```python
from build123d import *

# Parameters (mm, degrees)
F0_R     = 3.9751
F0_R_2   = 15.875
F0_R_3   = 3.96875
F1_DEPTH = 19.05
F3_DEPTH = 9.525
F5_R     = 9.525
F5_R_2   = 3.9751
F5_R_3   = 3.96875
F6_DEPTH = 2.54


# Not quite as in the source:
# - a feature of the source that left no trace in its solid (it failed there, or was rolled back) is left out


with BuildPart() as f1:
    # F0 (on Top) → F1 (new body)
    with BuildSketch(Plane.XY):
        with BuildLine():
            Line((-68.2625, -74.6125), (68.2625, -74.6125))
            ThreePointArc((68.2625, -74.6125), (72.7526280605, -72.7526280605), (74.6125, -68.2625))
            Line((74.6125, -68.2625), (74.6125, -4.7625))
            Line((74.6125, -4.7625), (15.1437848225, -4.7625))
            ThreePointArc((15.1437848225, -4.7625), (-15.875, 0), (15.1437848225, 4.7625))
            Line((15.1437848225, 4.7625), (74.6125, 4.7625))
            Line((74.6125, 4.7625), (74.6125, 68.2625))
            ThreePointArc((74.6125, 68.2625), (72.7526280605, 72.7526280605), (68.2625, 74.6125))
            Line((68.2625, 74.6125), (-68.2625, 74.6125))
            ThreePointArc((-68.2625, 74.6125), (-72.7526280605, 72.7526280605), (-74.6125, 68.2625))
            Line((-74.6125, 68.2625), (-74.6125, -68.2625))
            ThreePointArc((-74.6125, -68.2625), (-72.7526280605, -72.7526280605), (-68.2625, -74.6125))
        make_face()
        with Locations((-55.5625, -55.5625)):
            Circle(F0_R, mode=Mode.SUBTRACT)
        with Locations((-30.1625, -30.1625)):
            Circle(F0_R_2, mode=Mode.SUBTRACT)
        with Locations((55.5625, -55.5625)):
            Circle(F0_R, mode=Mode.SUBTRACT)
        with Locations((30.1625, -30.1625)):
            Circle(F0_R_2, mode=Mode.SUBTRACT)
        with Locations((-30.1625, 30.1625)):
            Circle(F0_R_2, mode=Mode.SUBTRACT)
        with Locations((-55.5625, 55.5625)):
            Circle(F0_R_3, mode=Mode.SUBTRACT)
        with Locations((30.1625, 30.1625)):
            Circle(F0_R_2, mode=Mode.SUBTRACT)
        with Locations((55.5625, 55.5625)):
            Circle(F0_R, mode=Mode.SUBTRACT)
    extrude(amount=F1_DEPTH)

    # F2 (on face) → F3 (join)
    with BuildSketch(Plane(origin=(0, 0, 0), x_dir=(1, 0, 0), z_dir=(0, 0, -1))):
        with BuildLine():
            Line((74.6125, 4.7625), (15.1437848225, 4.7625))
            ThreePointArc((15.1437848225, 4.7625), (15.875, 0), (15.1437848225, -4.7625))
            Line((15.1437848225, -4.7625), (74.6125, -4.7625))
            Line((74.6125, -4.7625), (74.6125, 4.7625))
        make_face()
    extrude(amount=-F3_DEPTH)

    # F5 (on face) → F6 (cut)
    with BuildSketch(Plane.XY.offset(19.05)):
        with Locations((-55.5625, -55.5625)):
            Circle(F5_R)
        with Locations((-55.5625, -55.5625)):
            Circle(F5_R_2, mode=Mode.SUBTRACT)
        with Locations((55.5625, -55.5625)):
            Circle(F5_R)
        with Locations((55.5625, -55.5625)):
            Circle(F5_R_2, mode=Mode.SUBTRACT)
        with Locations((55.5625, 55.5625)):
            Circle(F5_R)
        with Locations((55.5625, 55.5625)):
            Circle(F5_R_2, mode=Mode.SUBTRACT)
        with Locations((-55.5625, 55.5625)):
            Circle(F5_R)
        with Locations((-55.5625, 55.5625)):
            Circle(F5_R_3, mode=Mode.SUBTRACT)
    extrude(amount=-F6_DEPTH, mode=Mode.SUBTRACT)


solid = f1.part
```
Work out the finished part from the listing and answer in its coordinate system (mm). A direction names the side the tool comes from. Give positions to 0.01 mm unless a question says otherwise; leave off trailing zeros. Write item = value, one per line.
Q1. Flat-ended cylindrical pins translate along their axes: pin 1 Ø9 at (x, y) = (55.56, 55.56) entering from +Z; pin 2 Ø4 at (x, y) = (-39.5, -12) entering from -Z. Find the tip coordinate at first contact, or state that the pin passes through.
Computed values:
pin_1 = 16.51
pin_2 = 0
Q2. Section C-C on z = 3.5 is taken. State how many separate pieces and enclosed holes the cut face has, and give its area (3 significant figures).
Computed values:
separate_pieces = 1
enclosed_holes = 9
area = 18,100 mm^2
Q3. For a pull along Y with two mould halves and no side action, classify faces 1 (the flat face through (-1, -74.612, 9)), 2 (the cylindrical face through (18.46, 40.89, 9.39)), 3 (the flat face through (1, 74.612, 9)), 4 (the flat face through (-18, 1, 19.05)) as pulls with the +Y half, pulls with the -Y half, needs draft (parallel to the pull), parting line crosses it, or undercut.
Computed values:
face_1 = pulls with the -Y half
face_2 = undercut
face_3 = pulls with the +Y half
face_4 = needs draft
Q4. A tool of negligible diameter and unlimited length cuts with its end or side. For faces 5 (the flat face through (-51, 56, 16.51)), 6 (the flat face through (45, -4.762, 14)), 7 (the cylindrical face through (-72.703, 72.802, 9.392)), from which of +Z, -Z, +X, -X, +Y, -Y can it reach the whole face along a straight path? Write none if from no direction.
Computed values:
face_5 = +Z
face_6 = +Z, +X
face_7 = +Z, -Z, -X, +Y
Q5. Consider line 1 along Y through (x, z) = (31, 2.25); line 2 along X through (y, z) = (-56, 4.75); line 3 along X through (y, z) = (-30, 7.5). Determine where each line is inside the solid, lowest interval first.
Computed values:
line_1 = -74.61 to -46.02, -14.31 to 14.31, 46.02 to 74.61
line_2 = -74.61 to -59.51, -51.61 to 51.61, 59.51 to 74.61
line_3 = -74.61 to -46.04, -14.29 to 14.29, 46.04 to 74.61
